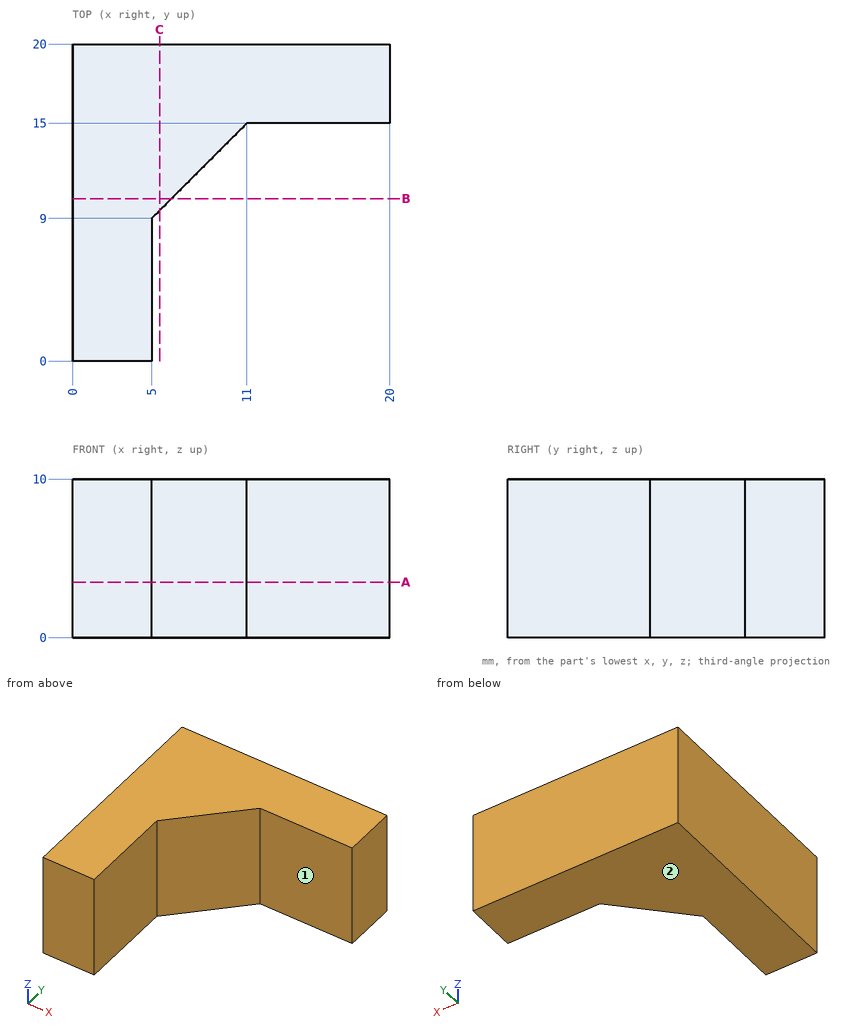
Design review of the part shown in the three views and the two pictorial views. Dimensions are in mm from the part's minimum x, y and z. A direction names the side the tool comes from. Round coordinates to 2 decimals unless told otherwise and drop trailing zeros. Write each loop counter-clockwise with the first axis right and the second up, starting at its lowest first coordinate (ties: lowest second). Pieces come first, ordered by that corner, then holes. Notation, with made-up numbers: (39, 2) -> (82, 2) arc R17 cw to (82, 23) -> close; hole circle Ø1 at (-28, -21). An arc over 180 degrees is marked (long way). Answer as a JSON object with one key per item and string values.
1. Machinability: for the marked faces 1 and 2, which of the approach directions +Z, -Z, +X, -X, +Y, -Y give a long, thin tool a straight path to every point of the face, cutting with its end or side? Answer none if there is none.
Results found:
{"face 1": "+Z, -Z, +X, -Y", "face 2": "-Z, +X, -X, +Y, -Y"}
2. To check wall thickness, follow line 1 along Y through (x, z) = (16, 8.25); line 2 along X through (y, z) = (13, 1.5); line 3 along X through (y, z) = (2, 5.5). State the ranges of each line that lie inside material, in increasing order.
Results found:
{"line 1": "y = 15 to 20", "line 2": "x = 0 to 9", "line 3": "x = 0 to 5"}
3. Clearance check with flat-ended pins moving along their axes: pin 1 (6 mm diameter, centred on y = 17.5, z = 2.5, fed in from -X); pin 2 (5 mm diameter, centred on x = 8.5, z = 2, fed in from -Y). State where each tip first meets the part, or that it passes through.
Results found:
{"pin 1": "stops at x = 0", "pin 2": "stops at y = 10"}
4. We need section A-A on z = 3.5. State the section outline as (x, y) points, and give its area (3 significant figures).
Results found:
{"outline": "(0, 0) -> (5, 0) -> (5, 9) -> (11, 15) -> (20, 15) -> (20, 20) -> (0, 20) -> close", "area": "193 mm^2"}
5. We need section B-B on y = 10.25. State the section outline as (x, z) points.
Results found:
{"outline": "(0, 0) -> (6.25, 0) -> (6.25, 10) -> (0, 10) -> close"}
6. We need section C-C on x = 5.5. State the section outline as (y, z) points.
Results found:
{"outline": "(9.5, 0) -> (20, 0) -> (20, 10) -> (9.5, 10) -> close"}
